Autodesk Inventor part; units mm, degrees
ref_plane "YZ Plane" through (0, 0, 0) normal (1, 0, 0) x (0, 1, 0)
ref_plane "XZ Plane" through (0, 0, 0) normal (0, 1, 0) x (-1, 0, 0)
ref_plane "XY Plane" through (0, 0, 0) normal (0, 0, 1) x (1, 0, 0)
sketch "Эскиз1" plane through (0, 0, 0) normal (0, 0, 1) x (1, 0, 0)
  circle A0 centre (0, 0) radius 135
  dimension "d0" = 270
extrude "Выдавливание1" add sketch "Эскиз1" along normal mid plane 6
sketch "Эскиз2" plane through (0, 0, 3) normal (0, 0, 1) x (1, 0, 0)
  circle A0 centre (0, 0) radius 120 construction
  line L0 (0, 0) -> (0, -223.6058) construction
  point P0 (0, -120)
  dimension "d3" = 240
hole "Отверстие1" at (0, -120, 3) direction (0, 0, -1) diameter 3.2 end through all
pattern_circular "Круговой массив1" count 4 over 360 about axis through (0, 0, 0) along (0, 0, 1) of "Отверстие1"
sketch "Эскиз3" plane through (0, 0, -3) normal (0, 0, -1) x (-1, 0, 0)
  circle A0 centre (0, 0) radius 50
  dimension "d14" = 100
extrude "Выдавливание2" cut sketch "Эскиз3" against normal through all
sketch "Эскиз4" plane through (0, 0, -3) normal (0, 0, -1) x (-1, 0, 0)
  circle A0 centre (44.8931, -30.0102) radius 2.25 construction
  point P0 (0, 0)
hole "Отверстие2" at (-44.8931, -30.0102, -3) direction (0, 0, 1) diameter 3.4 end through all
pattern_circular "Круговой массив2" count 6 over 360 about axis through (0, 0, -3) along (0, 0, 1) of "Отверстие2"
properties part number "Диск_опорный" material "По умолчанию1"
Geometry check sheet. Reference: the model listing, model coordinates, mm. Coordinates: 2 decimals unless noted, no trailing zeros. Write each loop counter-clockwise with the first axis right and the second up, starting at its lowest first coordinate (ties: lowest second). Pieces come first, ordered by that corner, then holes. Notation, with made-up numbers: M 82.5,72.25 L 94.5,72.25 A33 ccw 94.5,110.25 Z; hole C -24.75,3.25 d1. An arc over 180 degrees is marked long. Use one line per item in the form item = value. Start each with the question number.
1) Section check A-A on x = 26.5. Enter the section's corners in (y, z), and give its area (3 significant figures).
2) Section check C-C on y = -12. Enter the section's corners in (x, z).
3) Go/stop test with flat-tipped pins: pin 1 Ø2 at (x, y) = (-48.44, 23.87) entering from -Z; pin 2 Ø1.5 at (y, z) = (-97, -1.5) entering from -X. Record where each tip stops, or that it passes through.
4) Release check for a two-part mould opening along X. For faces 1 (the cylindrical face through (-47.69, 15.02, -0.04)), 2 (the flat face through (-2, -58, -3)), 3 (the cylindrical face through (-107.13, -82.15, 0.04)) record: pulls with the +X half, pulls with the -X half, needs draft (parallel to the pull), parting line crosses it, or undercut.
5) Thickness scan on probe 1 along Y at (x, z) = (-44.5, 0.1); probe 2 along Y at (x, z) = (-16.5, 1.7); probe 3 along Y at (x, z) = (12, -1.15). Record the ranges inside material, lowest first. Write a range as from..to.
6) Section check D-D on x = -56. Enter the section's corners in (y, z), and give its area (3 significant figures).
Responses:
q1.outline = M -132.37,-3 L -42.4,-3 L -42.4,3 L -132.37,3 Z; M 42.4,-3 L 132.37,-3 L 132.37,3 L 42.4,3 Z
q1.area = 1,080 mm2
q2.outline = M -134.47,-3 L -48.54,-3 L -48.54,3 L -134.47,3 Z; M 48.54,-3 L 134.47,-3 L 134.47,3 L 48.54,3 Z
q3.pin_1 = through
q3.pin_2 = -94.66
q4.face_1 = undercut
q4.face_2 = needs draft
q4.face_3 = parting line crosses it
q5.probe_1 = -127.45..-31.66, -28.36..-22.8, 22.8..127.45
q5.probe_2 = -133.99..-47.2, 47.2..133.99
q5.probe_3 = -134.47..-48.54, 48.54..134.47
q6.outline = M -122.84,-3 L 122.84,-3 L 122.84,3 L -122.84,3 Z
q6.area = 1,470 mm2
